Read the model definition and answer for the solid it produces. Units are mm, in the model's axes. Coordinates: 2 decimals unless noted, no trailing zeros. Write each loop counter-clockwise with the first axis right and the second up, starting at its lowest first coordinate (ties: lowest second). Pieces come first, ordered by that corner, then holes.
from build123d import *

# Parameters (mm, degrees)
BOSS_EXTRUDE1_DEPTH             = 120
SKETCH10_W                      = 2.5
SKETCH10_H                      = 10
F_5_0MM_DOWEL_HOLE1_AT_2_COUNT  = 2
F_5_0MM_DOWEL_HOLE1_AT_2_PITCH  = 230
F_5_0MM_DOWEL_HOLE1_AT_3_COUNT  = 2
F_5_0MM_DOWEL_HOLE1_AT_3_PITCH  = 250.79872408
F_5_0MM_DOWEL_HOLE1_AT_4_COUNT  = 2
F_5_0MM_DOWEL_HOLE1_AT_4_PITCH  = 152.397506541
F_5_0MM_DOWEL_HOLE1_AT_5_COUNT  = 2
F_5_0MM_DOWEL_HOLE1_AT_5_PITCH  = 100
F_5_0MM_DOWEL_HOLE1_AT_6_COUNT  = 2
F_5_0MM_DOWEL_HOLE1_AT_6_PITCH  = 115
SKETCH13_W                      = 5
SKETCH13_H                      = 20
F_10_0MM_DOWEL_HOLE1_AT_2_COUNT = 2
F_10_0MM_DOWEL_HOLE1_AT_2_PITCH = 115
F_10_0MM_DOWEL_HOLE1_AT_3_COUNT = 2
F_10_0MM_DOWEL_HOLE1_AT_3_PITCH = 230
F_10_0MM_DOWEL_HOLE1_AT_4_COUNT = 2
F_10_0MM_DOWEL_HOLE1_AT_4_PITCH = 250.79872408
F_10_0MM_DOWEL_HOLE1_AT_5_COUNT = 2
F_10_0MM_DOWEL_HOLE1_AT_5_PITCH = 152.397506541
F_10_0MM_DOWEL_HOLE1_AT_6_COUNT = 2
F_10_0MM_DOWEL_HOLE1_AT_6_PITCH = 100


with BuildPart() as part:
    # Sketch1 → Boss-Extrude1 (new body)
    with BuildSketch(Plane.XY):
        with BuildLine():
            Line((-20, 5), (4.406999064, 5))
            add(Edge.make_bspline(
                [(173.490575932, 5), (172.326342066, 5.286749118), (167.829693344, 6.405018282), (160.005568623, 8.421384221), (150.022959876, 10.929293239), (140.032690883, 13.242212873), (130.039576349, 15.224534417), (120.039677674, 16.776832577), (110.010328484, 17.519452934), (100.004268105, 17.93606864), (89.999557234, 18.039439262), (79.99597078, 17.88209955), (69.992122817, 17.447369698), (59.98803219, 16.737630926), (49.981633888, 15.747713143), (39.97167458, 14.434248174), (29.95037961, 12.743709227), (21.617032213, 10.901524907), (14.966560888, 9.053828582), (9.928778454, 7.425562721), (6.425978449, 5.993531691), (4.603660534, 5.099329751), (4.406999064, 5)],
                knots=[0.065553478, 0.065553478, 0.065553478, 0.065553478, 0.074294227, 0.099342978, 0.124359733, 0.149264719, 0.174009696, 0.198546974, 0.22290397, 0.247200686, 0.271477726, 0.295756352, 0.320054721, 0.344391349, 0.368786978, 0.393273071, 0.417900952, 0.442781229, 0.455381891, 0.468160436, 0.481314037, 0.482916031, 0.482916031, 0.482916031, 0.482916031], degree=3))
            Line((173.490575932, 5), (230, 5))
            Line((230, 5), (230, 35))
            Line((230, 35), (-20, 35))
            Line((-20, 35), (-20, 5))
        make_face()
    extrude(amount=BOSS_EXTRUDE1_DEPTH)

    # Sketch10 → Ø5.0mm Dowel Hole1 (revolve, cut)
    with BuildSketch(Plane(origin=(-10, 25, 10), x_dir=(0, 0, -1), z_dir=(1, 0, 0))):
        with Locations((1.25, 5)):
            Rectangle(SKETCH10_W, SKETCH10_H)
    f_5_0mm_dowel_hole1 = revolve(axis=Axis((-10, 18.65, 10), (0, 1, 0)), mode=Mode.SUBTRACT)

    # Ø5.0mm Dowel Hole1 at 2: Ø5.0mm Dowel Hole1 ×2
    with Locations(*[(i * F_5_0MM_DOWEL_HOLE1_AT_2_PITCH, 0, 0) for i in range(1, F_5_0MM_DOWEL_HOLE1_AT_2_COUNT)]):
        add(f_5_0mm_dowel_hole1, mode=Mode.SUBTRACT)

    # Ø5.0mm Dowel Hole1 at 3: Ø5.0mm Dowel Hole1 ×2
    with Locations(*[Vector(0.917070056253235, 0, 0.39872611141445) * (i * F_5_0MM_DOWEL_HOLE1_AT_3_PITCH) for i in range(1, F_5_0MM_DOWEL_HOLE1_AT_3_COUNT)]):
        add(f_5_0mm_dowel_hole1, mode=Mode.SUBTRACT)

    # Ø5.0mm Dowel Hole1 at 4: Ø5.0mm Dowel Hole1 ×2
    with Locations(*[Vector(0.7546055221635047, 0, 0.6561787149247866) * (i * F_5_0MM_DOWEL_HOLE1_AT_4_PITCH) for i in range(1, F_5_0MM_DOWEL_HOLE1_AT_4_COUNT)]):
        add(f_5_0mm_dowel_hole1, mode=Mode.SUBTRACT)

    # Ø5.0mm Dowel Hole1 at 5: Ø5.0mm Dowel Hole1 ×2
    with Locations(*[(0, 0, i * F_5_0MM_DOWEL_HOLE1_AT_5_PITCH) for i in range(1, F_5_0MM_DOWEL_HOLE1_AT_5_COUNT)]):
        add(f_5_0mm_dowel_hole1, mode=Mode.SUBTRACT)

    # Ø5.0mm Dowel Hole1 at 6: Ø5.0mm Dowel Hole1 ×2
    with Locations(*[(i * F_5_0MM_DOWEL_HOLE1_AT_6_PITCH, 0, 0) for i in range(1, F_5_0MM_DOWEL_HOLE1_AT_6_COUNT)]):
        add(f_5_0mm_dowel_hole1, mode=Mode.SUBTRACT)

    # Sketch13 → Ø10.0mm Dowel Hole1 (revolve, cut)
    with BuildSketch(Plane(origin=(-10, 25, 10), x_dir=(0, 0, 1), z_dir=(1, 0, 0))):
        with Locations((2.5, 10)):
            Rectangle(SKETCH13_W, SKETCH13_H)
    f_10_0mm_dowel_hole1 = revolve(axis=Axis((-10, 31.35, 10), (0, -1, 0)), mode=Mode.SUBTRACT)

    # Ø10.0mm Dowel Hole1 at 2: Ø10.0mm Dowel Hole1 ×2
    with Locations(*[(i * F_10_0MM_DOWEL_HOLE1_AT_2_PITCH, 0, 0) for i in range(1, F_10_0MM_DOWEL_HOLE1_AT_2_COUNT)]):
        add(f_10_0mm_dowel_hole1, mode=Mode.SUBTRACT)

    # Ø10.0mm Dowel Hole1 at 3: Ø10.0mm Dowel Hole1 ×2
    with Locations(*[(i * F_10_0MM_DOWEL_HOLE1_AT_3_PITCH, 0, 0) for i in range(1, F_10_0MM_DOWEL_HOLE1_AT_3_COUNT)]):
        add(f_10_0mm_dowel_hole1, mode=Mode.SUBTRACT)

    # Ø10.0mm Dowel Hole1 at 4: Ø10.0mm Dowel Hole1 ×2
    with Locations(*[Vector(0.917070056253235, 0, 0.39872611141445) * (i * F_10_0MM_DOWEL_HOLE1_AT_4_PITCH) for i in range(1, F_10_0MM_DOWEL_HOLE1_AT_4_COUNT)]):
        add(f_10_0mm_dowel_hole1, mode=Mode.SUBTRACT)

    # Ø10.0mm Dowel Hole1 at 5: Ø10.0mm Dowel Hole1 ×2
    with Locations(*[Vector(0.7546055221635047, 0, 0.6561787149247866) * (i * F_10_0MM_DOWEL_HOLE1_AT_5_PITCH) for i in range(1, F_10_0MM_DOWEL_HOLE1_AT_5_COUNT)]):
        add(f_10_0mm_dowel_hole1, mode=Mode.SUBTRACT)

    # Ø10.0mm Dowel Hole1 at 6: Ø10.0mm Dowel Hole1 ×2
    with Locations(*[(0, 0, i * F_10_0MM_DOWEL_HOLE1_AT_6_PITCH) for i in range(1, F_10_0MM_DOWEL_HOLE1_AT_6_COUNT)]):
        add(f_10_0mm_dowel_hole1, mode=Mode.SUBTRACT)


solid = part.part
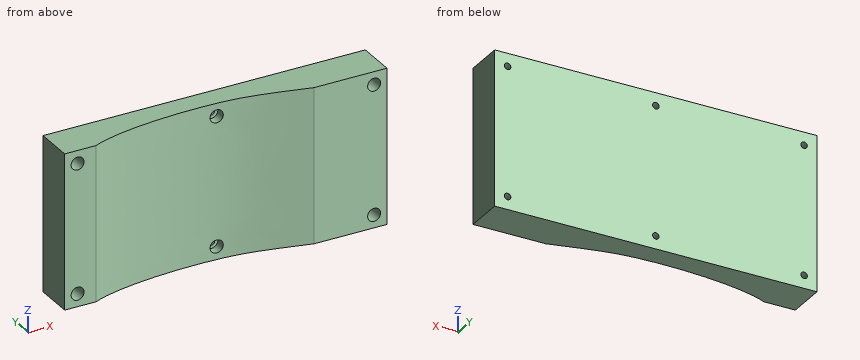
Item 1: The part is cut by section A-A (x = 220). Give the vertices of the cut face in (y, z).
Item 2: Given pin 1 (11 mm diameter, centred on x = 221.5, z = 12, fed in from -Y); pin 2 (6 mm diameter, centred on x = -10, z = 110, fed in from -Y); pin 3 (4 mm diameter, centred on x = 17.5, z = 18, fed in from -Y) (3 decimals); pin 4 (1 mm diameter, centred on x = 115, z = 40.5, fed in from -Y), each flat-ended and moving along its own axis, determine where each tip first touches the part or whether it passes through.
Item 3: The part is cut by section B-B (y = 11). State how many separate pieces and enclosed holes the cut face has, and give its area (3 significant figures).
Item 4: Find the intervals of material crossed by probe 1 along X at (y, z) = (30, 10); probe 2 along Z at (x, y) = (-10, 32); probe 3 along Z at (x, y) = (-10, 11), in increasing order.
Answer:
1. outline: (5, 0) - (35, 0) - (35, 7.5) - (25, 7.5) - (25, 5) - (5, 5) - close; (5, 15) - (25, 15) - (25, 12.5) - (35, 12.5) - (35, 107.5) - (25, 107.5) - (25, 105) - (5, 105) - close; (5, 115) - (25, 115) - (25, 112.5) - (35, 112.5) - (35, 120) - (5, 120) - close
2. pin 1: stops at y = 5
2. pin 2: stops at y = 25
2. pin 3: stops at y = 9.175
2. pin 4: stops at y = 17.09
3. separate pieces: 2
3. enclosed holes: 4
3. area: 14,400 mm2
4. probe 1: x = -20 to -12.5, -7.5 to 102.5, 107.5 to 217.5, 222.5 to 230
4. probe 2: z = 0 to 7.5, 12.5 to 107.5, 112.5 to 120
4. probe 3: z = 0 to 5, 15 to 105, 115 to 120
